from build123d import *

# Parameters (mm, degrees)
SKETCH1_R           = 2.413
BOSS_EXTRUDE1_DEPTH = 3.2004
SKETCH2_R           = 2.413
CUT_EXTRUDE1_DEPTH  = 3.2004
SKETCH5_R           = 1.7272
SKETCH5_W           = 40.894
SKETCH5_H           = 20.32
CUT_EXTRUDE3_DEPTH  = 149.410997158
SKETCH6_R           = 1.7272
CUT_EXTRUDE4_DEPTH  = 3.2004
SKETCH7_R           = 2.413
CUT_EXTRUDE5_DEPTH  = 3.2004
SKETCH8_R           = 1.7272
CUT_EXTRUDE6_DEPTH  = 3.2004


with BuildPart() as part:
    # Sketch1 → Boss-Extrude1 (new body)
    with BuildSketch(Plane.XY):
        with BuildLine():
            Line((120.015, 52.11572), (0, 52.11572))
            Line((0, 52.11572), (-15.54366081, 29.673353196))
            ThreePointArc((-15.54366081, 29.673353196), (-16.74897968, 10.134216365), (0, 0))
            Line((0, 0), (120.015, 0))
            ThreePointArc((120.015, 0), (136.76397968, 10.134216365), (135.55866081, 29.673353196))
            Line((135.55866081, 29.673353196), (120.015, 52.11572))
        make_face()
        with Locations((120.015, 18.90776)):
            Circle(SKETCH1_R, mode=Mode.SUBTRACT)
        with Locations((0, 18.90776)):
            Circle(SKETCH1_R, mode=Mode.SUBTRACT)
        with Locations((15.37290121, 18.90776)):
            Circle(SKETCH1_R, mode=Mode.SUBTRACT)
    extrude(amount=BOSS_EXTRUDE1_DEPTH)

    # Sketch2 → Cut-Extrude1 (cut)
    with BuildSketch(Plane(origin=(0, 0, 0), x_dir=(-1, 0, 0), z_dir=(0, 0, -1))):
        with Locations((-92.0115, 48.11522)):
            Circle(SKETCH2_R)
        with Locations((-76.0095, 48.11522)):
            Circle(SKETCH2_R)
        with Locations((-44.0055, 48.11522)):
            Circle(SKETCH2_R)
        with Locations((-28.0035, 48.11522)):
            Circle(SKETCH2_R)
    extrude(amount=-CUT_EXTRUDE1_DEPTH, mode=Mode.SUBTRACT)

    # Sketch5 → Cut-Extrude3 (cut, through all)
    with BuildSketch(Plane(origin=(0, 0, 0), x_dir=(-1, 0, 0), z_dir=(0, 0, -1))):
        with Locations((-73.48130308, 23.90776)):
            Circle(SKETCH5_R)
        with Locations((-22.98130308, 13.90776)):
            Circle(SKETCH5_R)
        with Locations((-22.98130308, 23.90776)):
            Circle(SKETCH5_R)
        with Locations((-73.48130308, 13.90776)):
            Circle(SKETCH5_R)
        with Locations((-48.23130308, 18.90776)):
            Rectangle(SKETCH5_W, SKETCH5_H)
    extrude(amount=-CUT_EXTRUDE3_DEPTH, mode=Mode.SUBTRACT)

    # Sketch6 → Cut-Extrude4 (cut)
    with BuildSketch(Plane.XY.offset(3.2004)):
        with Locations((97.03369692, 23.90776)):
            Circle(SKETCH6_R)
        with Locations((97.03369692, 13.90776)):
            Circle(SKETCH6_R)
        with BuildLine():
            Line((23.72030308, 19.92376), (27.78430308, 19.92376))
            Line((27.78430308, 19.92376), (27.78430308, 17.89176))
            Line((27.78430308, 17.89176), (23.72030308, 17.89176))
            ThreePointArc((23.72030308, 17.89176), (22.70430308, 18.90776), (23.72030308, 19.92376))
        make_face()
        with BuildLine():
            Line((68.67830308, 19.92376), (72.74230308, 19.92376))
            ThreePointArc((72.74230308, 19.92376), (73.75830308, 18.90776), (72.74230308, 17.89176))
            Line((72.74230308, 17.89176), (68.67830308, 17.89176))
            Line((68.67830308, 17.89176), (68.67830308, 19.92376))
        make_face()
    extrude(amount=-CUT_EXTRUDE4_DEPTH, mode=Mode.SUBTRACT)

    # Sketch7 → Cut-Extrude5 (cut)
    with BuildSketch(Plane(origin=(0, 0, 0), x_dir=(-1, 0, 0), z_dir=(0, 0, -1))):
        with Locations((-99.400822531, 30.809360911)):
            Circle(SKETCH7_R)
    extrude(amount=-CUT_EXTRUDE5_DEPTH, mode=Mode.SUBTRACT)

    # Sketch8 → Cut-Extrude6 (cut)
    with BuildSketch(Plane.XY.offset(3.2004)):
        with Locations((21.9075, 3.81)):
            Circle(SKETCH8_R)
        with Locations((60.0075, 3.81)):
            Circle(SKETCH8_R)
        with Locations((98.1075, 3.81)):
            Circle(SKETCH8_R)
    extrude(amount=-CUT_EXTRUDE6_DEPTH, mode=Mode.SUBTRACT)


solid = part.part
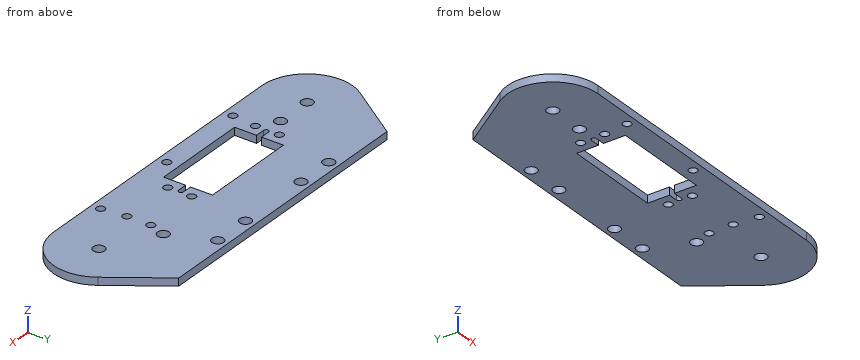
Work out the finished part from the listing and answer in its coordinate system (mm). Give positions to 0.01 mm unless a question says otherwise; leave off trailing zeros. Write each loop counter-clockwise with the first axis right and the second up, starting at its lowest first coordinate (ties: lowest second). Pieces come first, ordered by that corner, then holes. Notation, with made-up numbers: (-2.75, 84.5) - (38.25, 84.5) arc R26 ccw to (38.25, 99.5) - close; hole circle Ø10 at (64.25, 78). An arc over 180 degrees is marked (long way). One line per item, written item: value. Start each with the question number.
1. Find section A-A (y = 3.81). Write down the section's boundary in (x, z), then the cut area to 3 significant figures.
2. Find section C-C (y = 37.5). Write down the section's boundary in (x, z).
3. Find section B-B (z = 1.15). State how many separate pieces and enclosed holes the cut face has, then the cut area to 3 significant figures.
4. Consider probe 1 along Y at (x, z) = (69, 3.05); probe 2 along Y at (x, z) = (44, 1.55); probe 3 along X at (y, z) = (48.5, 1.9). Determine where each line is inside the solid, lowest interval first.
5. Given pin 1 (6.5 mm diameter, centred on x = 44.01, y = 48.12, fed in from -Z); pin 2 (1.6 mm diameter, centred on y = 12.5, z = 1, fed in from -X), each flat-ended and moving along its own axis, determine where each tip first touches the part or whether it passes through.
Geometry results:
1. outline: (-11.38, 0) - (20.18, 0) - (20.18, 3.2) - (-11.38, 3.2) - close; (23.63, 0) - (58.28, 0) - (58.28, 3.2) - (23.63, 3.2) - close; (61.73, 0) - (96.38, 0) - (96.38, 3.2) - (61.73, 3.2) - close; (99.83, 0) - (131.4, 0) - (131.4, 3.2) - (99.83, 3.2) - close
1. area: 424 mm2
2. outline: (-10.12, 0) - (130.14, 0) - (130.14, 3.2) - (-10.12, 3.2) - close
3. separate pieces: 1
3. enclosed holes: 18
3. area: 6,470 mm2
4. probe 1: 0 to 17.89, 19.92 to 52.12
4. probe 2: 0 to 8.75, 29.07 to 45.7, 50.53 to 52.12
4. probe 3: -2.5 to 25.62, 30.39 to 41.62, 46.39 to 73.63, 78.39 to 89.63, 94.39 to 122.52
5. pin 1: z = 0
5. pin 2: x = -18.06
